from build123d import *

# Parameters (mm, degrees)
SKETCH010_R     = 1.375
PAD005_DEPTH    = 1
FILLET001_R     = 1
PAD006_DEPTH    = 3
SKETCH012_W     = 57.5
SKETCH012_H     = 30.3
POCKET002_DEPTH = 0.2
SKETCH013_R     = 0.5
POCKET003_DEPTH = 4.001


with BuildPart() as part:
    # Sketch010 (on XY_Plane004 of Origin008) → Pad005 (new body)
    with BuildSketch(Plane.XY):
        Polygon((-35, -24.5), (-11, -24.5), (-11, -17.5), (0, -17.5), (11, -17.5), (11, -24.5), (35, -24.5), (35, 24.5), (-35, 24.5), align=None)
        with Locations((-32.725, 22.275)):
            Circle(SKETCH010_R, mode=Mode.SUBTRACT)
        with Locations((32.725, 22.275)):
            Circle(SKETCH010_R, mode=Mode.SUBTRACT)
        with Locations((-32.725, -21.225)):
            Circle(SKETCH010_R, mode=Mode.SUBTRACT)
        with Locations((32.725, -21.225)):
            Circle(SKETCH010_R, mode=Mode.SUBTRACT)
    extrude(amount=PAD005_DEPTH)

    # Fillet001
    fillet001_edges = [part.edges().sort_by_distance(p)[0] for p in [
        (-35, 24.5, 0.5),
        (35, 24.5, 0.5),
        (35, -24.5, 0.5),
        (-11, -17.5, 0.5),
        (-11, -24.5, 0.5),
        (11, -24.5, 0.5),
        (11, -17.5, 0.5),
        (-35, -24.5, 0.5),
    ]]
    fillet(fillet001_edges, radius=FILLET001_R)

    # Sketch011 (on Face2 of Fillet001) → Pad006 (join)
    with BuildSketch(Plane(origin=(0, 0, 0), x_dir=(1, 0, 0), z_dir=(0, 0, -1))):
        Polygon((-31.15, 18.7), (-31.15, -20.3), (31.15, -20.3), (31.15, 18.7), (19.15, 18.7), (18.15, 19.7), (-18.15, 19.7), (-19.15, 18.7), align=None)
    extrude(amount=PAD006_DEPTH)

    # Sketch012 (on Face32 of Pad006) → Pocket002 (cut)
    with BuildSketch(Plane(origin=(0, 0, -3), x_dir=(1, 0, 0), z_dir=(0, 0, -1))):
        with Locations((0, -3.15)):
            Rectangle(SKETCH012_W, SKETCH012_H)
    extrude(amount=-POCKET002_DEPTH, mode=Mode.SUBTRACT)

    # Sketch013 (on Face5 of Pocket002) → Pocket003 (cut, through all)
    with BuildSketch(Plane.XY.offset(1)):
        with Locations((33, -3.5)):
            Circle(SKETCH013_R)
        with Locations((33, -0.96)):
            Circle(SKETCH013_R)
        with Locations((33, 1.58)):
            Circle(SKETCH013_R)
        with Locations((33, 4.12)):
            Circle(SKETCH013_R)
    extrude(amount=-POCKET003_DEPTH, mode=Mode.SUBTRACT)


solid = part.part
The model under review builds one solid part; all positions refer to its coordinate system, in mm. A direction names the side the tool comes from. Give positions to 0.01 mm unless a question says otherwise; leave off trailing zeros. Write each loop counter-clockwise with the first axis right and the second up, starting at its lowest first coordinate (ties: lowest second). Pieces come first, ordered by that corner, then holes. Notation, with made-up numbers: M 88,62.5 L 144,62.5 A14 ccw 144,72.5 Z; hole C -40,-19.75 d10. An arc over 180 degrees is marked long. One line per question, with ' | ' between items. Start each with the question number.
Item 1: For faces 1 (the flat face through (0, -19, 0)), 2 (the flat face through (25, -18.7, -1)), 3 (the flat face through (-31.15, 1, -1)), 4 (the flat face through (0, 20.3, -1)), 5 (the flat face through (0, -19.7, -1)), list the 3-axis set-ups (+Z, -Z, +X, -X, +Y, -Y) from which the entire face can be reached by the end or side of a thin tool; tool diameter is ignored.
Item 2: Wall thickness on line 1 (X direction, y = 0, z = -1); line 2 (Z direction, x = 25, y = 6); line 3 (Y direction, x = 3, z = -0.75): over which ranges is each line inside the solid? List them lowest first. Write a range as from..to.
Item 3: We need section C-C on y = -8. Write out the cut boundary in (x, z), plus the area to 3 significant figures.
Item 4: We need section A-A on x = 24.5. Write out the cut boundary in (y, z).
Item 5: For pin 1 (2 mm diameter, centred on y = 5.5, z = -1.5, fed in from +X); pin 2 (3.5 mm diameter, centred on x = -32.725, y = 22.275, fed in from -Z); pin 3 (2 mm diameter, centred on x = -24.5, z = -2, fed in from +Y), all flat-tipped, find the tip position at first contact; note any pin that passes through.
Item 6: We need section B-B on z = -0.9. Write out the cut boundary in (x, y).
Item 7: Draft analysis for pull direction Y (two halves, no side actions). For faces 6 (the cylindrical face through (-31.455, -21.752, 0.493)), 7 (the flat face through (-25, -18.7, -1)), 8 (the flat face through (0, 0, 1)), state which applies: released by +Y, released by -Y, zero draft, split by the parting line, or undercut.
Results found:
1) face 1: +Z, -Y | face 2: -Z, +X, -Y | face 3: -Z, -X, +Y, -Y | face 4: -Z, +X, -X, +Y | face 5: -Z, +X, -X, -Y
2) line 1: x = -31.15..31.15 | line 2: z = -2.8..1 | line 3: y = -19.7..20.3
3) outline: M -35,0 L -31.15,0 L -31.15,-3 L -28.75,-3 L -28.75,-2.8 L 28.75,-2.8 L 28.75,-3 L 31.15,-3 L 31.15,0 L 35,0 L 35,1 L -35,1 Z | area: 245 mm2
4) outline: M -24.5,0 L -18.7,0 L -18.7,-3 L -12,-3 L -12,-2.8 L 18.3,-2.8 L 18.3,-3 L 20.3,-3 L 20.3,0 L 24.5,0 L 24.5,1 L -24.5,1 Z
5) pin 1: stops at x = 31.15 | pin 2: stops at z = 0 | pin 3: stops at y = 20.3
6) outline: M -31.15,-18.7 L -19.15,-18.7 L -18.15,-19.7 L 18.15,-19.7 L 19.15,-18.7 L 31.15,-18.7 L 31.15,20.3 L -31.15,20.3 Z
7) face 6: undercut | face 7: released by -Y | face 8: zero draft
